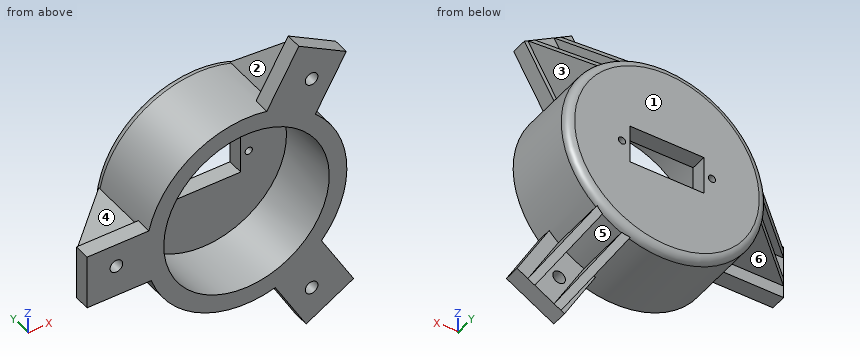
```python
from build123d import *

# Parameters (mm, degrees)
SKETCH1_R                   = 31.75
BOSS_EXTRUDE1_DEPTH         = 25.4
FILLET1_R                   = 2.54
SKETCH2_R                   = 26.178994306
CUT_EXTRUDE1_DEPTH          = 20.32
SKETCH3_W                   = 23.368
SKETCH3_H                   = 12.192
CUT_EXTRUDE2_DEPTH          = 20.32
SKETCH4_R                   = 1.143
CUT_EXTRUDE3_DEPTH          = 20.32
SKETCH6_W                   = 22.454622086
SKETCH6_H                   = 17.327996038
BOSS_EXTRUDE2_DEPTH         = 5.08
RIB1_REACH                  = 69.27
SKETCH11_WALL_W             = 162.351686776
SKETCH11_WALL_H             = 2.54
CIRPATTERN1_COUNT           = 3
CIRPATTERN1_COPY_1_REACH    = 69.27
CIRPATTERN1_COPY_1_SKETCH_W = 162.351686776
CIRPATTERN1_COPY_1_SKETCH_H = 2.54
CIRPATTERN1_COPY_2_REACH    = 69.27
CIRPATTERN1_COPY_2_SKETCH_W = 162.351686776
CIRPATTERN1_COPY_2_SKETCH_H = 2.54
SKETCH12_R                  = 2
CUT_EXTRUDE4_DEPTH          = 5.08
CIRPATTERN2_COUNT           = 3


with BuildPart() as part:
    # Sketch1 → Boss-Extrude1 (new body)
    with BuildSketch(Plane(origin=(0, 0, 0), x_dir=(1, 0, 0), z_dir=(0, 1, 0))):
        with Locations(Location((0, 0, 0), (0, 0, 270))):
            Circle(SKETCH1_R)
    extrude(amount=BOSS_EXTRUDE1_DEPTH)

    # Fillet1
    fillet1_edges = [part.edges().sort_by_distance(p)[0] for p in [
        (0, 25.4, -31.75),
    ]]
    fillet(fillet1_edges, radius=FILLET1_R)

    # Sketch2 → Cut-Extrude1 (cut)
    with BuildSketch(Plane.XZ):
        with Locations(Location((0, 0, 0), (0, 0, 270))):
            Circle(SKETCH2_R)
    extrude(amount=-CUT_EXTRUDE1_DEPTH, mode=Mode.SUBTRACT)

    # Sketch3 → Cut-Extrude2 (cut)
    with BuildSketch(Plane(origin=(0, 25.4, 0), x_dir=(1, 0, 0), z_dir=(0, 1, 0))):
        Rectangle(SKETCH3_W, SKETCH3_H)
    extrude(amount=-CUT_EXTRUDE2_DEPTH, mode=Mode.SUBTRACT)

    # Sketch4 → Cut-Extrude3 (cut)
    with BuildSketch(Plane(origin=(0, 25.4, 0), x_dir=(1, 0, 0), z_dir=(0, 1, 0))):
        with Locations(Location((-14.224, 0, 0), (0, 0, 270))):
            Circle(SKETCH4_R)
    cut_extrude3 = extrude(amount=-CUT_EXTRUDE3_DEPTH, mode=Mode.SUBTRACT)

    # Mirror1: Cut-Extrude3 across plane
    add(cut_extrude3.mirror(Plane(origin=(0, 0, 0), x_dir=(0, 0, 1), z_dir=(1, 0, 0))), mode=Mode.SUBTRACT)

    # Sketch6 → Boss-Extrude2 (add)
    with BuildSketch(Plane.XZ):
        with Locations((-39.218689259, -1.332922772)):
            Rectangle(SKETCH6_W, SKETCH6_H)
    boss_extrude2 = extrude(amount=-BOSS_EXTRUDE2_DEPTH)

    # Sketch11 wall → Rib1 (add, up to next)
    with BuildSketch(Plane(origin=(-41.089874413, 13.97, 4.791075247), x_dir=(0.724934415066, 0.688817896002, 0), z_dir=(-0.688817896002, 0.724934415066, 0)), mode=Mode.PRIVATE) as rib1_sk1:
        Rectangle(SKETCH11_WALL_W, SKETCH11_WALL_H)
    rib1_tool1 = extrude(rib1_sk1.sketch, amount=-RIB1_REACH, mode=Mode.PRIVATE) - part.part
    rib1 = rib1_tool1.solids().sort_by_distance((-41.089874413, 13.97, 4.791075247))[0]
    add(rib1)

    # Mirror2: Rib1 across plane
    add(rib1.mirror(Plane.XY))

    # CirPattern1: Boss-Extrude2, Rib1 ×3 about axis
    cirpattern1_axis = Axis((0, 0, 0), (0, 1, 0))
    add([boss_extrude2.rotate(cirpattern1_axis, i * 360 / CIRPATTERN1_COUNT) for i in range(1, CIRPATTERN1_COUNT)])
    add([rib1.rotate(cirpattern1_axis, i * 360 / CIRPATTERN1_COUNT) for i in range(1, CIRPATTERN1_COUNT)])

    # CirPattern1 copy 1 sketch → CirPattern1 copy 1 (add, up to next)
    with BuildSketch(Plane(origin=(16.395744331, 13.97, 37.980412703), x_dir=(-0.3624672075329998, 0.688817896002, -0.6278116195247685), z_dir=(0.34440894800099986, 0.724934415066, 0.5965337965190796)), mode=Mode.PRIVATE) as cirpattern1_copy_1_sk1:
        Rectangle(CIRPATTERN1_COPY_1_SKETCH_W, CIRPATTERN1_COPY_1_SKETCH_H)
    cirpattern1_copy_1_tool1 = extrude(cirpattern1_copy_1_sk1.sketch, amount=-CIRPATTERN1_COPY_1_REACH, mode=Mode.PRIVATE) - part.part
    add(cirpattern1_copy_1_tool1.solids().sort_by_distance((16.395744331, 13.97, 37.980412703))[0])

    # CirPattern1 copy 2 sketch → CirPattern1 copy 2 (add, up to next)
    with BuildSketch(Plane(origin=(24.694130082, 13.97, -33.189337456), x_dir=(-0.3624672075330003, 0.688817896002, 0.6278116195247683), z_dir=(0.34440894800100036, 0.724934415066, -0.5965337965190793)), mode=Mode.PRIVATE) as cirpattern1_copy_2_sk1:
        Rectangle(CIRPATTERN1_COPY_2_SKETCH_W, CIRPATTERN1_COPY_2_SKETCH_H)
    cirpattern1_copy_2_tool1 = extrude(cirpattern1_copy_2_sk1.sketch, amount=-CIRPATTERN1_COPY_2_REACH, mode=Mode.PRIVATE) - part.part
    add(cirpattern1_copy_2_tool1.solids().sort_by_distance((24.694130082, 13.97, -33.189337456))[0])

    # Sketch12 → Cut-Extrude4 (cut)
    with BuildSketch(Plane(origin=(0, 5.08, 0), x_dir=(1, 0, 0), z_dir=(0, 1, 0))):
        with Locations(Location((-41.1817754, 0, 0), (0, 0, 270))):
            Circle(SKETCH12_R)
    cut_extrude4 = extrude(amount=-CUT_EXTRUDE4_DEPTH, mode=Mode.SUBTRACT)

    # CirPattern2: Cut-Extrude4 ×3 about axis
    cirpattern2_axis = Axis((0, 0, 0), (0, 1, 0))
    for i in range(1, CIRPATTERN2_COUNT):
        add(cut_extrude4.rotate(cirpattern2_axis, i * 360 / CIRPATTERN2_COUNT), mode=Mode.SUBTRACT)


solid = part.part
```
Can you work these out from the model? Positions are in its coordinate system, mm. Face numbers are marked on the shaded views. A direction names the side the tool comes from. Round coordinates to 2 decimals unless told otherwise and drop trailing zeros. Order: outer loops, then holes, each group sorted by start corner. A loop starts at its lowest first (then second) coordinate and runs counter-clockwise, first axis right, second up. Notation, with made-up numbers: (46.5, 64.5) -> (73.5, 64.5) arc R10 cw to (73.5, 69.5) -> close; hole circle Ø6 at (45.25, 46.25). An arc over 180 degrees is marked (long way). Return JSON: item names as keys, results as strings. Group by question number.
1. If we section it at A-A, the plane x = 0: Write out the boundary of the cut face in (y, z).
2. If we section it at C-C, the plane z = 36.5: Write out the boundary of the cut face in (x, y), then the cut area to 3 significant figures.
3. If we section it at B-B, the plane z = 0: Write out the boundary of the cut face in (x, y).
4. We'd pull the mould along Z, two halves only. Please class the marked faces 1, 2 and 3: released by +Z, released by -Z, zero draft, split by the parting line, or undercut.
5. Will these pins go through, and if not, where does the flat tip stop? pin 1 (12 mm diameter, centred on x = 16.5, y = 11.5, fed in from +Z); pin 2 (4 mm diameter, centred on x = 10, z = 43, fed in from +Y); pin 3 (12 mm diameter, centred on y = 13.5, z = -29.5, fed in from -X); pin 4 (1.5 mm diameter, centred on x = 1.5, y = 22.5, fed in from +Z).
6. Which directions (+Z, -Z, +X, -X, +Y, -Y) give clear straight access to the entire face, cutting with the end or side of a thin tool? Please do the marked faces 4, 5 and 6.
7. I need wall thicknesses on line 1 (X direction, y = 4.5, z = 0); line 2 (X direction, y = 21.8, z = 0); line 3 (Z direction, x = -41.5, y = 3.25). Which ranges of each line are inside material? Lowest first, please. Write a range as [from, to].
Output values:
{
 "1": {"outline": "(0, -31.75) -> (22.86, -31.75) arc R2.54 ccw to (25.4, -29.21) -> (25.4, -6.1) -> (20.32, -6.1) -> (20.32, -26.18) -> (0, -26.18) -> close; (0, 26.18) -> (20.32, 26.18) -> (20.32, 6.1) -> (25.4, 6.1) -> (25.4, 29.21) arc R2.54 ccw to (22.86, 31.75) -> (0, 31.75) -> close"},
 "2": {"outline": "(9.53, 0) -> (18.77, 0) -> (18.77, 5.08) -> (17.01, 5.08) -> (17.01, 14.9) -> (14.07, 16.29) -> (14.07, 5.08) -> (9.53, 5.08) -> close; (22.41, 0) -> (29.54, 0) -> (29.54, 5.08) -> (28.07, 5.08) -> (28.07, 9.64) -> (25.14, 11.03) -> (25.14, 5.08) -> (22.41, 5.08) -> close", "area": "129 mm²"},
 "3": {"outline": "(-50.45, 0) -> (-43.18, 0) -> (-43.18, 5.08) -> (-50.45, 5.08) -> close; (-39.18, 0) -> (-26.18, 0) -> (-26.18, 20.32) -> (-15.37, 20.32) -> (-15.37, 25.4) -> (-29.21, 25.4) arc R2.54 ccw to (-31.75, 22.86) -> (-31.75, 5.08) -> (-39.18, 5.08) -> close; (-13.08, 20.32) -> (-11.68, 20.32) -> (-11.68, 25.4) -> (-13.08, 25.4) -> close; (11.68, 20.32) -> (13.08, 20.32) -> (13.08, 25.4) -> (11.68, 25.4) -> close; (15.37, 20.32) -> (26.18, 20.32) -> (26.18, 0) -> (31.75, 0) -> (31.75, 22.86) arc R2.54 ccw to (29.21, 25.4) -> (15.37, 25.4) -> close"},
 "4": {"face 1": "zero draft", "face 2": "released by +Z", "face 3": "undercut"},
 "5": {"pin 1": "z = 45.67", "pin 2": "through", "pin 3": "x = -21.35", "pin 4": "z = 31.74"},
 "6": {"face 4": "+Z, -X, +Y", "face 5": "+Y", "face 6": "-Z, -X, +Y"},
 "7": {"line 1": "[-50.45, -43.18], [-39.18, -26.18], [26.18, 31.75]", "line 2": "[-31.75, -15.37], [-13.08, -11.68], [11.68, 13.08], [15.37, 31.75]", "line 3": "[-10, -1.97], [1.97, 7.33]"}
}
